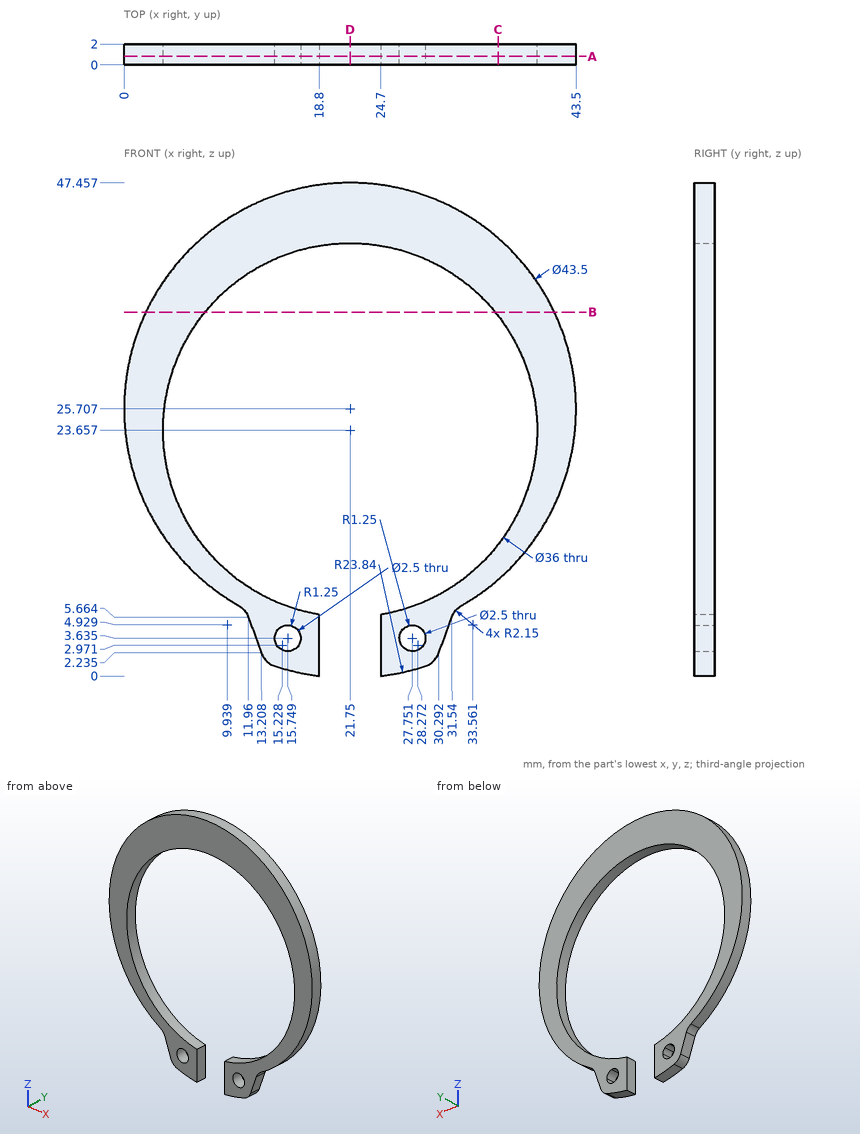
For this review, use the dimensioned drawing (mm, ordinates from the lowest corner) and the shaded views. Give positions to 0.01 mm unless a question says otherwise; leave off trailing zeros. Loops run counter-clockwise (first coordinate to the right, second up) from the corner with the lowest first, then second, coordinate; pieces in that order, holes last.
Item 1: Insertion check: pin 1 (6 mm diameter, centred on x = 33, z = 31.5, fed in from +Y); pin 2 (0.6 mm diameter, centred on y = 1, z = 2, fed in from -X); pin 3 (3.5 mm diameter, centred on x = 15.75, z = 3.64, fed in from +Y). Each pin has a flat end and moves straight along its axis. Give the tip position at first contact, or say it passes through.
Item 2: Take a section at A-A, the plane y = 0.8. Give the number of separate pieces and of enclosed holes in the cut face.
Item 3: For line 1 along Z through (x, y) = (33.5, 1.4) (1 decimal); line 2 along X through (y, z) = (1.15, 10.5) (1 decimal); line 3 along X through (y, z) = (1.55, 23.5), list the stretches that pass through material, from the lowest coordinate up.
Item 4: Take a section at B-B, the plane z = 35. State the section outline as (x, y) points (1 decimal).
Item 5: Take a section at C-C, the plane x = 36. State the section outline as (y, z) points (1 decimal).
Item 6: Take a section at D-D, the plane x = 21.75. State the section outline as (y, z) points, and give its area (3 significant figures).
Calculated:
1. pin 1: passes through
1. pin 2: stops at x = 13.18
1. pin 3: stops at y = 2
2. separate pieces: 1
2. enclosed holes: 2
3. line 1: z = 7.4 to 10, 37.3 to 44
3. line 2: x = 6.2 to 9.5, 34 to 37.3
3. line 3: x = 0.11 to 3.75, 39.75 to 43.39
4. outline: (2.1, 0) - (7.8, 0) - (7.8, 2) - (2.1, 2) - close; (35.7, 0) - (41.4, 0) - (41.4, 2) - (35.7, 2) - close
5. outline: (0, 9.3) - (2, 9.3) - (2, 12.7) - (0, 12.7) - close; (0, 34.7) - (2, 34.7) - (2, 42.1) - (0, 42.1) - close
6. outline: (0, 41.66) - (2, 41.66) - (2, 47.46) - (0, 47.46) - close
6. area: 11.6 mm2
